Geometry check sheet. Reference: the model listing, model coordinates, mm. Face numbers are marked on the shaded views. A direction names the side the tool comes from. Coordinates: 2 decimals unless noted, no trailing zeros. Order: outer loops, then holes, each group sorted by start corner. A loop starts at its lowest first (then second) coordinate and runs counter-clockwise, first axis right, second up. Notation, with made-up numbers: (28.25, -37.75) - (64.25, -37.75) arc R27 ccw to (64.25, -6.75) - close; hole circle Ø11 at (11.25, 69.25). An arc over 180 degrees is marked (long way). One line per item, written item: value. Start each with the question number.
```python
from build123d import *

# Parameters (mm, degrees)
F1_DEPTH  = 101.6
F3_DEPTH  = 100.0125
F4_R      = 5.08
F5_R      = 5.08
F6_R      = 8.636
F7_DEPTH  = 25.4
F9_DEPTH  = 25.4
F10_W     = 25.4
F10_H     = 63.5
F11_DEPTH = 25.4
F13_DEPTH = 0.79375


with BuildPart() as f1:
    # F0 (on Top) → F1 (new body)
    with BuildSketch(Plane.XY):
        with BuildLine():
            ThreePointArc((0, -17.4625), (12.347852, -12.347852), (17.4625, 0))
            ThreePointArc((17.4625, 0), (12.347852, 12.347852), (0, 17.4625))
            ThreePointArc((0, 17.4625), (-17.4625, 0), (0, -17.4625))
        make_face()
        with BuildLine():
            Line((17.4625, -17.4625), (17.4625, 0))
            ThreePointArc((17.4625, 0), (12.347852, -12.347852), (0, -17.4625))
            Line((0, -17.4625), (17.4625, -17.4625))
        make_face()
        with BuildLine():
            ThreePointArc((0, 17.4625), (12.347852, 12.347852), (17.4625, 0))
            Line((17.4625, 0), (17.4625, 17.4625))
            Line((17.4625, 17.4625), (0, 17.4625))
        make_face()
    extrude(amount=F1_DEPTH)

    # F2 (on face) → F3 (cut)
    with BuildSketch(Plane.XY.offset(101.6)):
        with BuildLine():
            ThreePointArc((0, -15.875), (11.22532, -11.22532), (15.875, 0))
            ThreePointArc((15.875, 0), (11.22532, 11.22532), (0, 15.875))
            ThreePointArc((0, 15.875), (-15.875, 0), (0, -15.875))
        make_face()
        with BuildLine():
            Line((15.875, -15.875), (15.875, 0))
            ThreePointArc((15.875, 0), (11.22532, -11.22532), (0, -15.875))
            Line((0, -15.875), (15.875, -15.875))
        make_face()
        with BuildLine():
            ThreePointArc((0, 15.875), (11.22532, 11.22532), (15.875, 0))
            Line((15.875, 0), (15.875, 15.875))
            Line((15.875, 15.875), (0, 15.875))
        make_face()
    extrude(amount=-F3_DEPTH, mode=Mode.SUBTRACT)

    # F4
    f4_edges = [f1.edges().sort_by_distance(p)[0] for p in [
        (17.4625, -17.4625, 50.8),
        (17.4625, 17.4625, 50.8),
    ]]
    fillet(f4_edges, radius=F4_R)

    # F5
    f5_edges = [f1.edges().sort_by_distance(p)[0] for p in [
        (15.875, 15.875, 51.59375),
        (15.875, -15.875, 51.59375),
    ]]
    fillet(f5_edges, radius=F5_R)

    # F6 (on face) → F7 (cut)
    with BuildSketch(Plane.YZ.offset(17.4625)):
        with Locations((0, 87.3125)):
            Circle(F6_R)
    extrude(amount=-F7_DEPTH, mode=Mode.SUBTRACT)

    # F8 (on face) → F9 (cut)
    with BuildSketch(Plane.YZ.offset(17.4625)):
        Polygon((-3.96875, 5.08), (0, 5.08), (3.96875, 5.08), (3.96875, 17.78), (-3.96875, 17.78), align=None)
    extrude(amount=-F9_DEPTH, mode=Mode.SUBTRACT)

    # F10 (on Right) → F11 (cut)
    with BuildSketch(Plane.YZ):
        with Locations((0, 38.1)):
            Rectangle(F10_W, F10_H)
    extrude(amount=-F11_DEPTH, mode=Mode.SUBTRACT)

    # F12 (on face) → F13 (cut)
    with BuildSketch(Plane.XY.offset(1.5875)):
        with BuildLine():
            Line((6.35, 11.1125), (-4.7625, 11.1125))
            ThreePointArc((-4.7625, 11.1125), (-15.875, 0), (-4.7625, -11.1125))
            Line((-4.7625, -11.1125), (6.35, -11.1125))
            Line((6.35, -11.1125), (6.35, 11.1125))
        make_face()
    extrude(amount=-F13_DEPTH, mode=Mode.SUBTRACT)


solid = f1.part
```
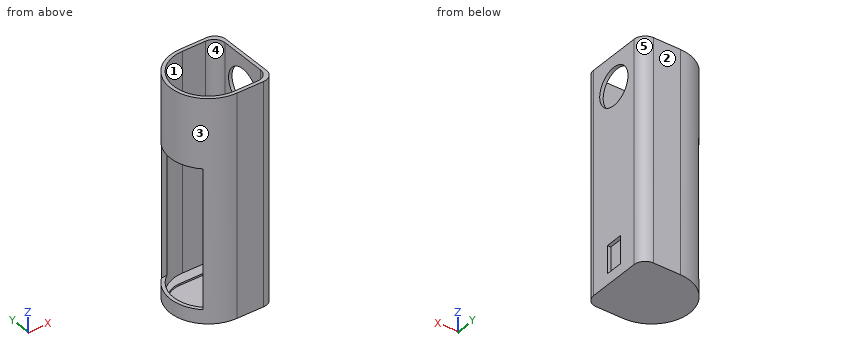
Q1. Gauge pin test, flat ends, axial feed: P1, Ø0.8, axis at x = 16.5, z = 11, coming from the -Y side; P2, Ø3, axis at x = -8.5, z = 16.5, coming from the +Y side; P3, Ø1.2, axis at x = -10.5, z = 34.5, coming from the -Y side (3 decimals). Record the tip position at first contact, or that the pin passes through.
Q2. Release check for a two-part mould opening along Y. For the marked faces 3, 4 and 5 record: released by +Y, released by -Y, zero draft, split by the parting line, or undercut.
Q3. Cross-section at B-B, the plane x = 9.5. Enter the section's corners in (y, z) (1 decimal).
Q4. Set-up check for the marked faces 1 and 2: record each of +Z, -Z, +X, -X, +Y, -Y from which the full face is reachable in a straight line by a thin tool's end or side.
Q5. Cross-section at D-D, the plane x = -14. Enter the section's corners in (y, z), and give its area (3 significant figures).
Q6. Material ranges on probe 1 along Z at (x, y) = (16.9, 0); probe 2 along Z at (x, y) = (-16, -4.5); probe 3 along Y at (x, z) = (8, 64) (1 decimal), recorded low to high.
Q7. Cross-section at A-A, the plane y = 7.5. Count the separate pieces of the cut face and the enclosed holes in it, and give its area (3 significant figures).
Check result:
1. P1: stops at y = -15.84
1. P2: stops at y = 16
1. P3: stops at y = -14.385
2. face 3: split by the parting line
2. face 4: undercut
2. face 5: released by +Y
3. outline: (-17.5, 0) - (17.5, 0) - (17.5, 101.6) - (15.9, 101.6) - (15.9, 1.6) - (-15.9, 1.6) - (-15.9, 101.6) - (-17.5, 101.6) - close
4. face 1: +Z
4. face 2: +Z, -Z, +X, -X, +Y
5. outline: (-10.44, 0) - (10.44, 0) - (10.44, 6.35) - (7.48, 6.35) - (7.48, 1.59) - (6.18, 1.59) - (6.18, 0.79) - (-6.18, 0.79) - (-6.18, 1.59) - (-7.48, 1.59) - (-7.48, 6.35) - (-10.44, 6.35) - close; (-10.44, 69.85) - (-7.48, 69.85) - (-7.48, 101.6) - (-10.44, 101.6) - close; (7.48, 69.85) - (10.44, 69.85) - (10.44, 101.6) - (7.48, 101.6) - close
5. area: 239 mm2
6. probe 1: z = 0 to 5.08, 17.78 to 78.68, 95.95 to 101.6
6. probe 2: z = 0 to 6.35, 69.85 to 101.6
6. probe 3: y = -17.5 to -15.9, 15.9 to 17.5
7. separate pieces: 3
7. enclosed holes: 0
7. area: 248 mm2
